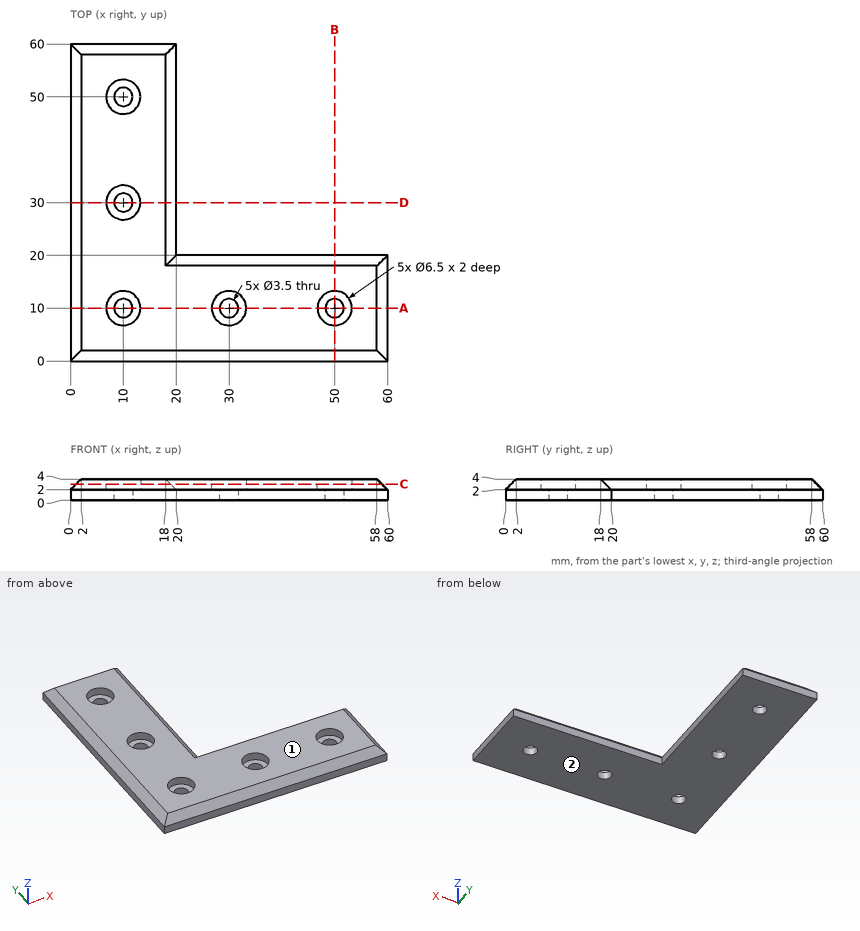
Answer from the drawing. Dimensions are ordinates in mm from the lowest x, y and z of the part. Coordinates: 2 decimals unless noted, no trailing zeros. Order: outer loops, then holes, each group sorted by start corner. A loop starts at its lowest first (then second) coordinate and runs counter-clockwise, first axis right, second up. Notation, with made-up numbers: (85.25, -16) - (96.25, -16) arc R36 ccw to (96.25, 21) - close; hole circle Ø6 at (-16.75, -29). An arc over 180 degrees is marked (long way). Use one line per item in the form item = value.
(1) Given pin 1 Ø1 at (x, z) = (48, 0.5) entering from +Y; pin 2 Ø4.5 at (x, y) = (30, 10) entering from +Z; pin 3 Ø1.5 at (y, z) = (43, 2.5) entering from +X, each flat-ended and moving along its own axis, determine where each tip first touches the part or whether it passes through.
Computed values:
pin_1 = 20
pin_2 = 2
pin_3 = 20
(2) For a pull along Z with two mould halves and no side action, classify the marked faces 1 and 2 as pulls with the +Z half, pulls with the -Z half, needs draft (parallel to the pull), parting line crosses it, or undercut.
Computed values:
face_1 = pulls with the +Z half
face_2 = pulls with the -Z half
(3) Section B-B, the plane x = 50 is taken. Give the vertices of the cut face in (y, z).
Computed values:
outline = (0, 0) - (8.25, 0) - (8.25, 2) - (6.75, 2) - (6.75, 4) - (2, 4) - (0, 2) - close; (11.75, 0) - (20, 0) - (20, 2) - (18, 4) - (13.25, 4) - (13.25, 2) - (11.75, 2) - close
(4) Section A-A, the plane y = 10 is taken. Give the number of separate pieces and of enclosed holes in the cut face, then the cut area to 3 significant figures.
Computed values:
separate_pieces = 4
enclosed_holes = 0
area = 176 mm²
(5) Straight lines are drawn through the part: L1, parallel to Y at x = 10, z = 1.5; L2, parallel to X at y = 9, z = 3.4; L3, parallel to Y at x = 10, z = 3.45. For each, find the intervals that lie inside material, in ascending order.
Computed values:
L1 = 0 to 8.25, 11.75 to 28.25, 31.75 to 48.25, 51.75 to 60
L2 = 1.4 to 6.91, 13.09 to 26.91, 33.09 to 46.91, 53.09 to 58.6
L3 = 1.45 to 6.75, 13.25 to 26.75, 33.25 to 46.75, 53.25 to 58.55
(6) Section C-C, the plane z = 3.05 is taken. Give the vertices of the cut face in (x, y).
Computed values:
outline = (1.05, 1.05) - (58.95, 1.05) - (58.95, 18.95) - (18.95, 18.95) - (18.95, 58.95) - (1.05, 58.95) - close; hole circle Ø6.5 at (10, 10); hole circle Ø6.5 at (10, 30); hole circle Ø6.5 at (10, 50); hole circle Ø6.5 at (30, 10); hole circle Ø6.5 at (50, 10)
